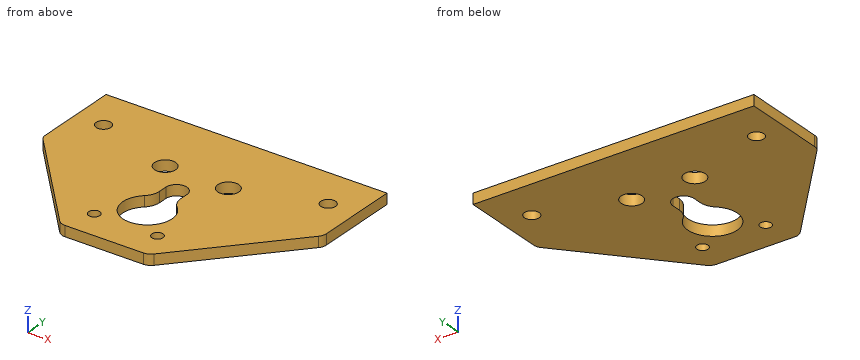
from build123d import *

# Parameters (mm, degrees)
SKETCH2_R           = 7
SKETCH2_R_2         = 1.6
BOSS_EXTRUDE1_DEPTH = 3
SKETCH3_R           = 2.1
CUT_EXTRUDE1_DEPTH  = 10
FILLET1_R           = 3
SKETCH4_R           = 3
CUT_EXTRUDE2_DEPTH  = 10
FILLET2_R           = 5


with BuildPart() as part:
    # Sketch2 → Boss-Extrude1 (new body)
    with BuildSketch(Plane.XY):
        Polygon((-12.5, -17), (12.5, -17), (40, 14), (40, 39), (-40, 39), (-40, 14), align=None)
        Circle(SKETCH2_R, mode=Mode.SUBTRACT)
        with Locations((-9, -8.5)):
            Circle(SKETCH2_R_2, mode=Mode.SUBTRACT)
        with Locations((9, -8.5)):
            Circle(SKETCH2_R_2, mode=Mode.SUBTRACT)
    extrude(amount=BOSS_EXTRUDE1_DEPTH)

    # Sketch3 → Cut-Extrude1 (cut)
    with BuildSketch(Plane.XY.offset(3)):
        with Locations((31.999, 26.93)):
            Circle(SKETCH3_R)
        with Locations((-31.999, 26.93)):
            Circle(SKETCH3_R)
    extrude(amount=-CUT_EXTRUDE1_DEPTH, mode=Mode.SUBTRACT)

    # Fillet1
    fillet1_edges = [part.edges().sort_by_distance(p)[0] for p in [
        (-40, 14, 1.5),
        (40, 14, 1.5),
        (12.5, -17, 1.5),
        (-12.5, -17, 1.5),
    ]]
    fillet(fillet1_edges, radius=FILLET1_R)

    # Sketch4 → Cut-Extrude2 (cut)
    with BuildSketch(Plane.XY.offset(3)):
        with Locations((9, 19.4)):
            Circle(SKETCH4_R)
        with Locations((-9, 19.4)):
            Circle(SKETCH4_R)
        with BuildLine():
            Line((-3, 11.4), (-3, 6.32455532))
            ThreePointArc((-3, 6.32455532), (0, 7), (3, 6.32455532))
            Line((3, 6.32455532), (3, 11.4))
            ThreePointArc((3, 11.4), (0, 14.4), (-3, 11.4))
        make_face()
    extrude(amount=-CUT_EXTRUDE2_DEPTH, mode=Mode.SUBTRACT)

    # Fillet2
    fillet2_edges = [part.edges().sort_by_distance(p)[0] for p in [
        (-3, 6.32455532, 1.5),
        (3, 6.32455532, 1.5),
    ]]
    fillet(fillet2_edges, radius=FILLET2_R)


solid = part.part
Verification items for the finished model (mm, model axes). Round coordinates to 2 decimals unless told otherwise and drop trailing zeros. Loops run counter-clockwise (first coordinate to the right, second up) from the corner with the lowest first, then second, coordinate; pieces in that order, holes last. Notation, with made-up numbers: (60, 12) - (72, 12) arc R19 ccw to (72, 47) - close; hole circle Ø11 at (-39, 19). An arc over 180 degrees is marked (long way). Use a Markdown table: item, result. Add a question column.
1. Thickness scan on probe 1 along Y at (x, z) = (-9, 0.3); probe 2 along X at (y, z) = (-9.5, 0.7); probe 3 along X at (y, z) = (25.5, 1.95). Record the ranges inside material, lowest first. Write a range as [from, to].
2. Gauge pin test, flat ends, axial feed: pin 1 (1.2 mm diameter, centred on y = 10, z = 1, fed in from +X); pin 2 (8 mm diameter, centred on x = -9, y = 19.4, fed in from +Z); pin 3 (2.5 mm diameter, centred on x = 31.999, y = 26.93, fed in from +Z). Record the tip position at first contact, or that the pin passes through.
3. Section check D-D, the plane z = 2. Record the boundary of the cut face in (x, y), plus the area to 3 significant figures.
4. Section check A-A, the plane x = 9. Record the boundary of the cut face in (y, z).
5. Section check B-B, the plane x = 0. Record the boundary of the cut face in (y, z), plus the area to 3 significant figures.
6. Section check C-C, the plane y = 26.93. Record the boundary of the cut face in (x, z).
Checks:
| question | item | result |
|---|---|---|
| 1 | probe 1 | y = [-17, -10.1], [-6.9, 16.4], [22.4, 39] |
| 1 | probe 2 | x = [-19.15, -10.25], [-7.75, 7.75], [10.25, 19.15] |
| 1 | probe 3 | x = [-40, -33.54], [-30.46, 30.46], [33.54, 40] |
| 2 | pin 1 | stops at x = 36.98 |
| 2 | pin 2 | stops at z = 3 |
| 2 | pin 3 | passes through |
| 3 | outline | (-40, 15.14) arc R3 ccw to (-39.24, 13.15) - (-13.4, -15.99) arc R3 ccw to (-11.15, -17) - (11.15, -17) arc R3 ccw to (13.4, -15.99) - (39.24, 13.15) arc R3 ccw to (40, 15.14) - (40, 39) - (-40, 39) - close; hole circle Ø4.2 at (-32, 26.93); hole circle Ø6 at (-9, 19.4); hole circle Ø3.2 at (-9, -8.5); hole (-4.67, 5.22) arc R7 ccw (long way) to (4.67, 5.22) arc R5 cw to (3, 8.94) - (3, 11.4) arc R3 ccw to (-3, 11.4) - (-3, 8.94) arc R5 cw to start; hole circle Ø6 at (9, 19.4); hole circle Ø3.2 at (9, -8.5); hole circle Ø4.2 at (32, 26.93) |
| 3 | area | 3,330 mm^2 |
| 4 | outline | (-17, 0) - (-10.1, 0) - (-10.1, 3) - (-17, 3) - close; (-6.9, 0) - (16.4, 0) - (16.4, 3) - (-6.9, 3) - close; (22.4, 0) - (39, 0) - (39, 3) - (22.4, 3) - close |
| 5 | outline | (-17, 0) - (-7, 0) - (-7, 3) - (-17, 3) - close; (14.4, 0) - (39, 0) - (39, 3) - (14.4, 3) - close |
| 5 | area | 104 mm^2 |
| 6 | outline | (-40, 0) - (-34.1, 0) - (-34.1, 3) - (-40, 3) - close; (-29.9, 0) - (29.9, 0) - (29.9, 3) - (-29.9, 3) - close; (34.1, 0) - (40, 0) - (40, 3) - (34.1, 3) - close |
